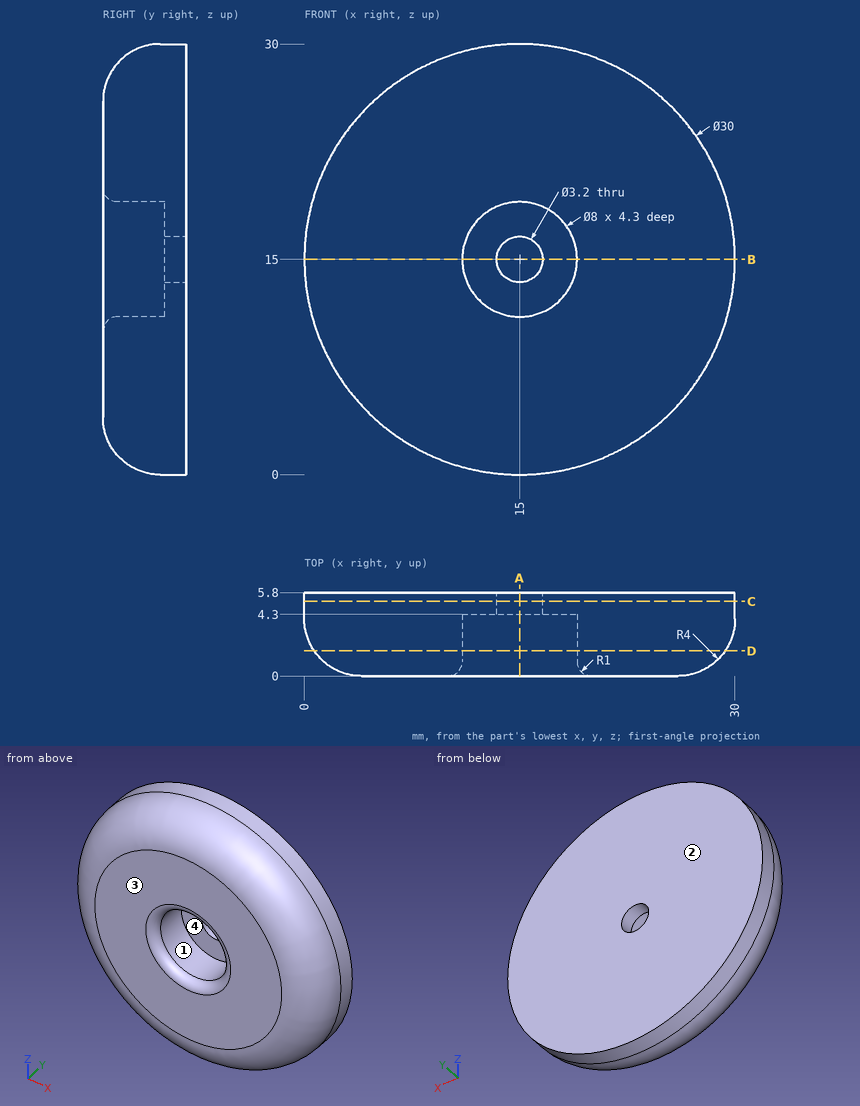
Answer from the drawing. Dimensions are ordinates in mm from the lowest x, y and z of the part. A direction names the side the tool comes from. Give positions to 0.01 mm unless a question says otherwise; leave off trailing zeros. Write each loop counter-clockwise with the first axis right and the second up, starting at its lowest first coordinate (ties: lowest second). Pieces come first, ordered by that corner, then holes.
1) A tool of negligible diameter and unlimited length cuts with its end or side. For the marked faces 3 and 4, from which of +Z, -Z, +X, -X, +Y, -Y can it reach the whole face along a straight path? Write none if from no direction.
2) Section A-A (x = 15) is taken. Write down the section's boundary in (y, z), and give its area (3 significant figures).
3) Section D-D (y = 1.75) is taken. Write down the section's boundary in (x, z), and give its area (3 significant figures).
4) For a pull along Z with two mould halves and no side action, classify the marked faces 1 and 2 as pulls with the +Z half, pulls with the -Z half, needs draft (parallel to the pull), parting line crosses it, or undercut.
5) Find the intervals of material crossed by L1, parallel to X at y = 4.1, z = 16.5; L2, parallel to Z at x = 15, y = 2.45; L3, parallel to X at y = 2.1, z = 28, in increasing order.
6) Section B-B (z = 15) is taken. Write down the section's boundary in (x, y).
7) Given P1, Ø1, axis at x = 20.5, y = 4.5, coming from the +Z side; P2, Ø2.5, axis at x = 15, z = 15, coming from the -Y side; P3, Ø1, axis at x = 9.5, z = 26, coming from the -Y side; P4, Ø1.5, axis at x = 11, y = 2, coming from the -Z side, each flat-ended and moving along its own axis, determine where each tip first touches the part or whether it passes through.
8) Section C-C (y = 5.2) is taken. Write down the section's boundary in (x, z), and give its area (3 significant figures).
Response:
1. face 3: +Z, -Z, +X, -X, -Y
1. face 4: -Y
2. outline: (0, 4) arc R4 ccw to (4, 0) - (5.8, 0) - (5.8, 13.4) - (4.3, 13.4) - (4.3, 11) - (1, 11) arc R1 ccw to (0, 10) - close; (0, 20) arc R1 ccw to (1, 19) - (4.3, 19) - (4.3, 16.6) - (5.8, 16.6) - (5.8, 30) - (4, 30) arc R4 ccw to (0, 26) - close
2. area: 128 mm2
3. outline: circle Ø28.61 at (15, 15); hole circle Ø8 at (15, 15)
3. area: 593 mm2
4. face 1: undercut
4. face 2: needs draft
5. L1: x = 0.08 to 11.29, 18.71 to 29.92
5. L2: z = 0.31 to 11, 19 to 29.69
5. L3: x = 8.53 to 21.47
6. outline: (0, 4) arc R4 ccw to (4, 0) - (10, 0) arc R1 ccw to (11, 1) - (11, 4.3) - (13.4, 4.3) - (13.4, 5.8) - (0, 5.8) - close; (16.6, 4.3) - (19, 4.3) - (19, 1) arc R1 ccw to (20, 0) - (26, 0) arc R4 ccw to (30, 4) - (30, 5.8) - (16.6, 5.8) - close
7. P1: stops at z = 29.14
7. P2: passes through
7. P3: stops at y = 0.08
7. P4: stops at z = 0.69
8. outline: circle Ø30 at (15, 15); hole circle Ø3.2 at (15, 15)
8. area: 699 mm2
